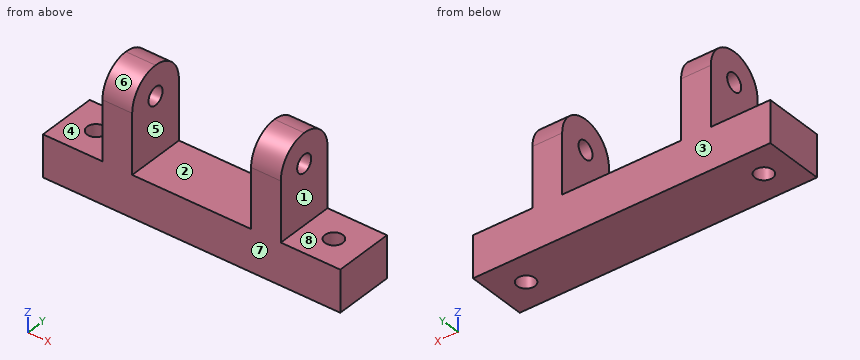
```python
from build123d import *

# Parameters (mm, degrees)
F0_W      = 50
F0_H      = 10
F1_DEPTH  = 7
F2_W      = 30
F2_H      = 10
F4_DEPTH  = 15
F5_R      = 4.99999
F3_R      = 1.5
F6_DEPTH  = 25
F7_R      = 1.5
F8_DEPTH  = 50
F10_W     = 20
F10_H     = 10
F11_DEPTH = 25


# Not quite as in the source:
# - a fillet or chamfer is up to 0.001 mm smaller than in the source, because OpenCascade refuses the exact size


with BuildPart() as f1:
    # F0 (on Top) → F1 (new body)
    with BuildSketch(Plane.XY):
        with Locations((25, 5)):
            Rectangle(F0_W, F0_H)
    extrude(amount=F1_DEPTH)

    # F2 (on face) → F4 (join)
    with BuildSketch(Plane.XY.offset(7)):
        with Locations((25, 5)):
            Rectangle(F2_W, F2_H)
    extrude(amount=F4_DEPTH)

    # F5 (radius 5 in the source; OpenCascade refuses exactly that, so slightly less here)
    f5_edges = [f1.edges().sort_by_distance(p)[0] for p in [
        (25, 10, 22),
        (25, 0, 22),
    ]]
    fillet(f5_edges, radius=F5_R)

    # F3 (on face) → F6 (cut)
    with BuildSketch(Plane.XY.offset(7)):
        with Locations((45, 5)):
            Circle(F3_R)
        with Locations((5, 5)):
            Circle(F3_R)
    extrude(amount=-F6_DEPTH, mode=Mode.SUBTRACT)

    # F7 (on face) → F8 (cut)
    with BuildSketch(Plane.YZ.offset(40)):
        with Locations((5, 17)):
            Circle(F7_R)
    extrude(amount=-F8_DEPTH, mode=Mode.SUBTRACT)


with BuildPart() as f9_1:
    # F9: copy of F1
    add(f1.part.moved(Location((0, 0, 40))))

    # F10 (on face) → F11 (cut)
    with BuildSketch(Plane.XY.offset(47)):
        with Locations((25, 5)):
            Rectangle(F10_W, F10_H)
    extrude(amount=F11_DEPTH, mode=Mode.SUBTRACT)


solid = f9_1.part
```
Can you work these out from the model? Positions are in its coordinate system, mm. Face numbers are marked on the shaded views. A direction names the side the tool comes from. Round coordinates to 2 decimals unless told otherwise and drop trailing zeros. Order: outer loops, then holes, each group sorted by start corner. A loop starts at its lowest first (then second) coordinate and runs counter-clockwise, first axis right, second up.
(1) If we section it at A-A (x = 45): Please give me the cut outline in (y, z).
Results are:
outline: (0, 40) - (3.5, 40) - (3.5, 47) - (0, 47) - close; (6.5, 40) - (10, 40) - (10, 47) - (6.5, 47) - close
(2) If we section it at B-B (z = 48): Please give me the cut outline in (x, y).
Results are:
outline: (10, 0) - (15, 0) - (15, 10) - (10, 10) - close; (35, 0) - (40, 0) - (40, 10) - (35, 10) - close
(3) On a 3-axis mill with a long thin cutter (end or side, diameter ignored), from which of +Z, -Z, +X, -X, +Y, -Y can I reach the whole of each face in a straight line? I mean the marked faces 4, 5, 6, 7 and 8. Say none if no direction works.
Results are:
face 4: +Z, -X, +Y, -Y
face 5: +Z, +Y, -Y
face 6: +Z, +X, -X, -Y
face 7: +Z, -Z, +X, -X, -Y
face 8: +Z, +X, +Y, -Y
(4) I'm going to push flat-ended pins straight in: pin 1 (3 mm diameter, centred on x = 45, y = 7, fed in from +Z); pin 2 (5 mm diameter, centred on y = 7.5, z = 50, fed in from -X); pin 3 (3 mm diameter, centred on y = 7.5, z = 52, fed in from +X). Where does each tip first touch, or does it pass through?
Results are:
pin 1: stops at z = 47
pin 2: stops at x = 10
pin 3: stops at x = 40
(5) If I drill on L1, parallel to X at y = 2.5, z = 53.5; L2, parallel to Z at x = 36.4, y = 5; L3, parallel to Y at x = 5, z = 41.75, over which ranges is the centre line in solid material (lowest first)?
Results are:
L1: x = 10 to 15, 35 to 40
L2: z = 40 to 55.5, 58.5 to 62
L3: y = 0 to 3.5, 6.5 to 10
(6) If we section it at D-D (z = 45.5): Please give me the cut outline in (x, y), plus the area to 3 significant figures.
Results are:
outline: (0, 0) - (50, 0) - (50, 10) - (0, 10) - close; hole circle Ø3 at (5, 5); hole circle Ø3 at (45, 5)
area: 486 mm2
(7) We'd pull the mould along X, two halves only. Please class the marked faces 1, 2 and 3: +X half, -X half, draft (parallel to the pull), parting line (faces both ways), or undercut.
Results are:
face 1: +X half
face 2: undercut
face 3: draft
